Can you work these out from the drawing? Everything is in mm from the part's minimum corner. A direction names the side the tool comes from. Give positions to 0.01 mm unless a question says otherwise; leave off trailing zeros. Order: outer loops, then holes, each group sorted by start corner. A loop starts at its lowest first (then second) coordinate and runs counter-clockwise, first axis right, second up. Notation, with made-up numbers: (18.25, 48.25) - (66.25, 48.25) arc R15 cw to (66.25, 74.25) - close; hole circle Ø11 at (34.25, 66.25). An arc over 180 degrees is marked (long way). One line per question, with ' | ' between items.
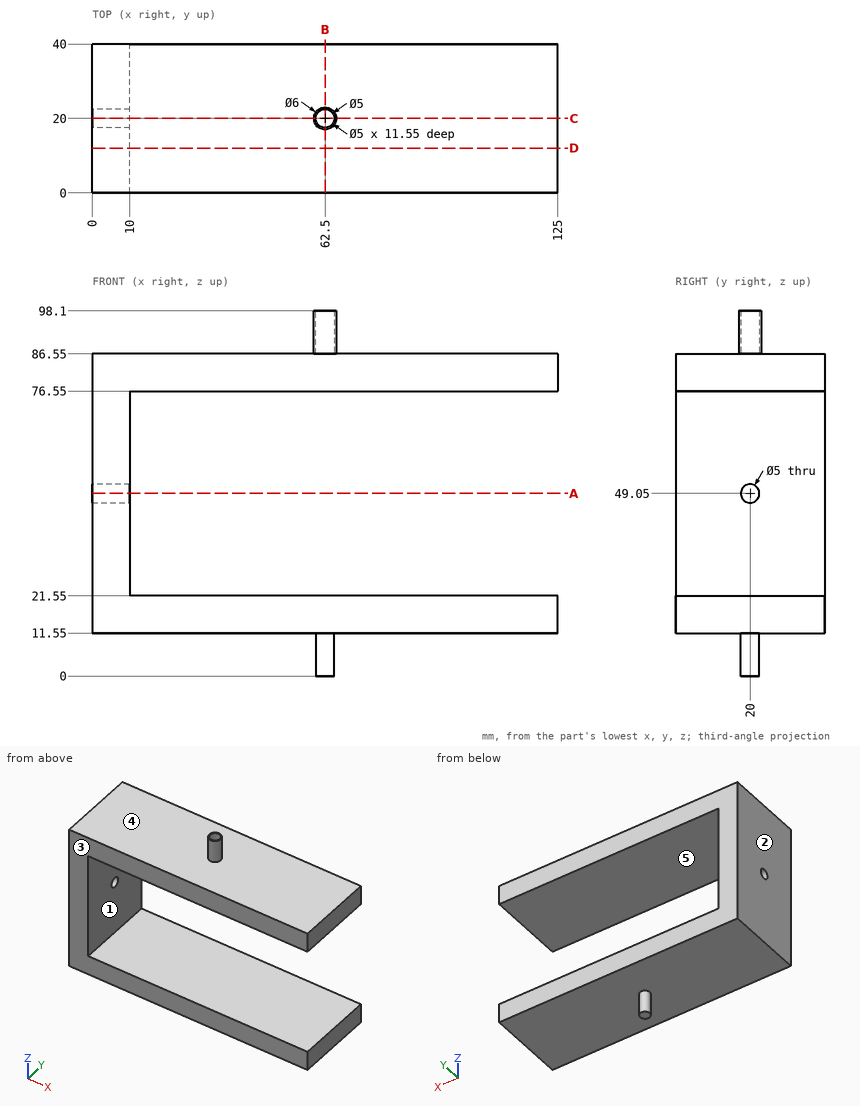
1) Thinking about a two-plate mould opening in Z: for the marked faces 3, 4 and 5, which applies, +Z half, -Z half, draft (parallel to the pull), parting line (faces both ways), or undercut?
Model answer:
face 3: draft | face 4: +Z half | face 5: undercut
2) I want a section at A-A (z = 49.05). List the corners of the cut face in (x, y) for me, plus the area to 3 significant figures.
Model answer:
outline: (0, 0) - (10, 0) - (10, 17.5) - (0, 17.5) - close; (0, 22.5) - (10, 22.5) - (10, 40) - (0, 40) - close | area: 350 mm2
3) I want a section at D-D (y = 12). List the corners of the cut face in (x, z) for me.
Model answer:
outline: (0, 11.55) - (125, 11.55) - (125, 21.55) - (10, 21.55) - (10, 76.55) - (125, 76.55) - (125, 86.55) - (0, 86.55) - close
4) On a 3-axis mill with a long thin cutter (end or side, diameter ignored), from which of +Z, -Z, +X, -X, +Y, -Y can I reach the whole of each face in a straight line? I mean the marked faces 1 and 2. Say none if no direction works.
Model answer:
face 1: +X, +Y, -Y | face 2: +Z, -Z, -X, +Y, -Y
5) Please list where these lines run through material, in increasing order: L1, parallel to Z at x = 90.5, y = 37.5; L2, parallel to Y at x = 62.5, z = 90.5; L3, parallel to X at y = 19.5, z = 37.5.
Model answer:
L1: z = 11.55 to 21.55, 76.55 to 86.55 | L2: y = 17 to 17.5, 22.5 to 23 | L3: x = 0 to 10
6) I want a section at C-C (y = 20). List the corners of the cut face in (x, z) for me, plus the area to 3 significant figures.
Model answer:
outline: (0, 11.55) - (60, 11.55) - (60, 0) - (65, 0) - (65, 11.55) - (125, 11.55) - (125, 21.55) - (10, 21.55) - (10, 46.55) - (0, 46.55) - close; (0, 51.55) - (10, 51.55) - (10, 76.55) - (125, 76.55) - (125, 86.55) - (65.5, 86.55) - (65.5, 98.1) - (65, 98.1) - (65, 86.55) - (60, 86.55) - (60, 98.1) - (59.5, 98.1) - (59.5, 86.55) - (0, 86.55) - close | area: 3,070 mm2
7) I want a section at B-B (x = 62.5). List the corners of the cut face in (y, z) for me.
Model answer:
outline: (0, 11.55) - (17.5, 11.55) - (17.5, 0) - (22.5, 0) - (22.5, 11.55) - (40, 11.55) - (40, 21.55) - (0, 21.55) - close; (0, 76.55) - (40, 76.55) - (40, 86.55) - (23, 86.55) - (23, 98.1) - (22.5, 98.1) - (22.5, 86.55) - (17.5, 86.55) - (17.5, 98.1) - (17, 98.1) - (17, 86.55) - (0, 86.55) - close
8) I'm going to push flat-ended pins straight in: P1, Ø8, axis at x = 29, y = 7, coming from the +Z side; P2, Ø1, axis at y = 31, z = 42, coming from the -X side; P3, Ø12, axis at y = 21, z = 29, coming from the +X side; P4, Ø4, axis at x = 30.5, y = 31, coming from the -Z side. Where does each tip first touch, or does it pass through?
Model answer:
P1: stops at z = 86.55 | P2: stops at x = 0 | P3: stops at x = 10 | P4: stops at z = 11.55
